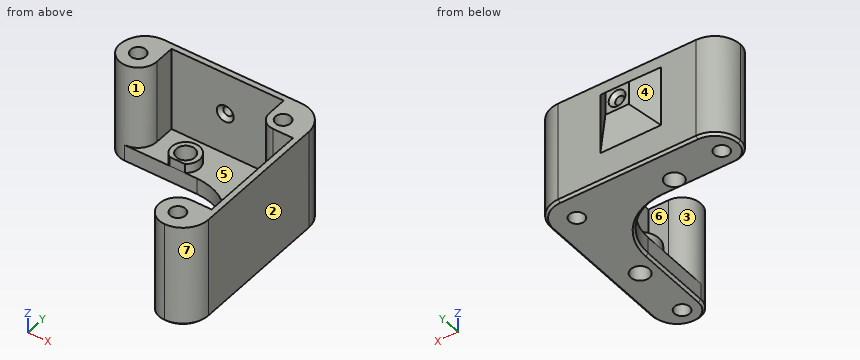
Solid Edge part; units mm, degrees
sketch "Sketch1" plane through (0, 0, 0) normal (0, 0, 1) x (1, 0, 0)
  line L0 (11.5, 0) -> (11.5, -15.5)
  arc A0 (11.5, -15.5) -> (15.5, -19.5) centre (15.5, -15.5) ccw
  arc A1 (15.5, -19.5) -> (21, -14) centre (15.5, -14) ccw
  line L1 (21, -14) -> (21, 15.5)
  arc A2 (21, 15.5) -> (15.5, 21) centre (15.5, 15.5) ccw
  line L2 (15.5, 21) -> (-14, 21)
  arc A3 (-19.5, 15.5) -> (-14, 21) centre (-14, 15.5) cw
  arc A4 (-15.5, 11.5) -> (-19.5, 15.5) centre (-15.5, 15.5) cw
  line L3 (0, 11.5) -> (-15.5, 11.5)
  arc A5 (0, 11.5) -> (11.5, 0) centre (0, 0) cw
extrude "Protrusion1" add sketch "Sketch1" along normal blind 22
sketch "Sketch2" plane through (0.75, 0.75, 22) normal (0, 0, 1) x (1, 0, 0)
  line L0 (-0.75, 10.75) -> (-16.25, 10.75)
  arc A0 (-16.25, 10.75) -> (-12.25, 14.75) centre (-16.25, 14.75) ccw
  line L1 (-12.25, 14.75) -> (-12.25, 19.05)
  line L2 (-12.25, 19.05) -> (11.75, 19.05)
  line L3 (11.75, 19.05) -> (11.75, 14.75)
  arc A1 (14.75, 11.75) -> (11.75, 14.75) centre (14.75, 14.75) cw
  line L4 (19.05, 11.75) -> (14.75, 11.75)
  line L5 (19.05, 11.75) -> (19.05, -12.25)
  line L6 (14.75, -12.25) -> (19.05, -12.25)
  arc A2 (10.75, -16.25) -> (14.75, -12.25) centre (14.75, -16.25) cw
  line L7 (10.75, -0.75) -> (10.75, -16.25)
  arc A3 (-0.75, 10.75) -> (10.75, -0.75) centre (-0.75, -0.75) cw
extrude "VaciadoExtruido_1" cut sketch "Sketch2" against normal blind 18
sketch "Sketch3" plane through (0, 0, 0) normal (0, 0, 1) x (1, 0, 0)
  circle A0 centre (-15.5, 15.5) radius 1.625
  circle A1 centre (15.5, 15.5) radius 1.625
  circle A2 centre (15.5, -15.5) radius 1.625
extrude "Cutout1" cut sketch "Sketch3" along normal through all
sketch "Sketch4" plane through (0.75, 21, 10.5) normal (0, 1, 0) x (-1, 0, 0)
  line L0 (-1.75, 0) -> (3.25, 0)
  line L1 (3.25, 0) -> (3.25, 5)
  line L2 (3.25, 5) -> (-1.75, 5)
  line L3 (-1.75, 5) -> (-1.75, 0)
extrude "ProtrusiónExtruida_2" add sketch "Sketch4" along normal blind 4
chamfer "Chaflán_1" distance 4 angle 45 4 edges at (-2.5, 21, 13) (0, 21, 15.5) (0, 21, 10.5) (2.5, 21, 13)
sketch "Sketch5" plane through (0.5, 19.8, 12) normal (0, -1, 0) x (1, 0, 0)
  circle A0 centre (-0.5, 1) radius 1
extrude "Cutout2" cut sketch "Sketch5" against normal through all
chamfer "Chaflán_2" distance 0.8 angle 45 2 edges at (0, 25, 12) (-1, 19.8, 13)
sketch "Sketch6" plane through (0.75, 0.75, 0) normal (0, 0, -1) x (1, 0, 0)
  line L0 (-6.6583, -10.75) -> (-3.3417, -10.75)
  arc A0 (-3.3417, -10.75) -> (-6.6583, -10.75) centre (-5, -13.25) cw
  circle A1 centre (14.75, 3.9) radius 4
extrude "Protrusion2" add sketch "Sketch6" against normal blind 6
sketch "Sketch7" plane through (0.75, 0.75, 0) normal (0, 0, -1) x (1, 0, 0)
  circle A0 centre (-5, -13.25) radius 2
  circle A1 centre (14.75, 3.9) radius 2
extrude "Cutout3" cut sketch "Sketch7" against normal through all
chamfer "Chaflán_4" distance 0.5 angle 45 10 edges at (8.1317, 8.1317, 0) (11.5, -7.75, 0) (12.6716, -18.3284, 0) (19.3891, -17.8891, 0) (21, 0.75, 0) (19.3891, 19.3891, 0) (0.75, 21, 0) (-17.8891, 19.3891, 0) (-18.3284, 12.6716, 0) (-7.75, 11.5, 0)
Design review of the part built by this model. Coordinates are the model's own, in mm. Face numbers are marked on the shaded views. A direction names the side the tool comes from. Coordinates: 2 decimals unless noted, no trailing zeros. Write each loop counter-clockwise with the first axis right and the second up, starting at its lowest first coordinate (ties: lowest second). Pieces come first, ordered by that corner, then holes. Notation, with made-up numbers: (11.5, 35) -> (69.5, 35) arc R20 cw to (69.5, 45) -> close; hole circle Ø8 at (22.25, -4.75). An arc over 180 degrees is marked (long way). Write each question's results on one line, items separated by ' | '. Start each with the question number.
(1) Take a section at C-C on y = 22. Write out the cut boundary in (x, z), and give its area (3 significant figures).
(2) For line 1 along X through (y, z) = (-3.15, 4.5); line 2 along Y through (x, z) = (15.5, 12) (3 decimals); line 3 along X through (y, z) = (-3.15, 3.5), list the stretches that pass through material, from the lowest coordinate up. Write a range as from..to.
(3) Take a section at A-A on z = 13. Give the number of separate pieces and of enclosed holes in the cut face, and give its area (3 significant figures).
(4) Tool access review of the marked faces 5, 6 and 7: name each direction out of +Z, -Z, +X, -X, +Y, -Y from which nothing blocks a thin tool from reaching the whole face with its end or side.
(5) The part is to be moulded in two halves that separate along Y. For the marked faces 1, 2, 3 and 4, say which applies: pulls with the +Y half, pulls with the -Y half, needs draft (parallel to the pull), parting line crosses it, or undercut.
(6) Take a section at D-D on x = -10. Write out the cut boundary in (y, z).
(7) Clearance check with flat-ended pins moving along their axes: P1, Ø9, axis at x = 15, y = -4, coming from the +Z side; P2, Ø2, axis at y = 18, z = 13, coming from the +X side; P3, Ø5.5, axis at y = 3, z = 12.5, coming from the -X side. State where each tip first meets the part, or that it passes through.
(8) Take a section at B-B on z = 1.5. Write out the cut boundary in (x, y) (3 decimals), and give its area (3 significant figures).
Results found:
1) outline: (-5.5, 7.5) -> (5.5, 7.5) -> (5.5, 18.5) -> (-5.5, 18.5) -> close; hole circle Ø2 at (0, 13) | area: 118 mm2
2) line 1: x = 11.5..13.5, 17.5..19.5, 19.8..21 | line 2: y = -19.5..-17.125, -13.875..-11.5, 12.5..13.875, 17.125..21 | line 3: x = 11.5..13.5, 17.5..21
3) separate pieces: 2 | enclosed holes: 3 | area: 246 mm2
4) face 5: +Z | face 6: +Z, -X | face 7: +Z, -Z, +X, -Y
5) face 1: pulls with the -Y half | face 2: needs draft | face 3: undercut | face 4: pulls with the +Y half
6) outline: (11.5, 0.5) -> (12, 0) -> (20.5, 0) -> (21, 0.5) -> (21, 22) -> (19.8, 22) -> (19.8, 4) -> (11.5, 4) -> close
7) P1: stops at z = 6 | P2: stops at x = 20.79 | P3: stops at x = 19.8
8) outline: (-19.5, 15.5) arc R4 ccw to (-15.5, 11.5) -> (0, 11.5) arc R11.5 cw to (11.5, 0) -> (11.5, -15.5) arc R4 ccw to (15.5, -19.5) arc R5.5 ccw to (21, -14) -> (21, 15.5) arc R5.5 ccw to (15.5, 21) -> (-14, 21) arc R5.5 ccw to start; hole circle Ø3.25 at (-15.5, 15.5); hole circle Ø4 at (-4.25, 14); hole circle Ø4 at (15.5, -3.15); hole circle Ø3.25 at (15.5, -15.5); hole circle Ø3.25 at (15.5, 15.5) | area: 631 mm2
